Autodesk Inventor part; units mm, degrees
ref_plane "Work Plane1" through (0, 0, 20) normal (0, 0, 1) x (1, 0, 0)
ref_plane "YZ Plane" through (0, 0, 0) normal (1, 0, 0) x (0, 1, 0)
ref_plane "XZ Plane" through (0, 0, 0) normal (0, 1, 0) x (-1, 0, 0)
sketch "Sketch1" plane through (0, 0, 0) normal (0, 0, 1) x (1, 0, 0)
  line L0 (-50, 0) -> (-50, 70)
  line L1 (-50, 70) -> (-115, 70)
  line L2 (-115, 70) -> (-115, 210)
  line L3 (-115, 210) -> (-75, 210)
  line L4 (-75, 210) -> (-75, 120)
  line L5 (-75, 120) -> (75, 120)
  line L6 (75, 120) -> (75, 210)
  line L7 (75, 210) -> (115, 210)
  line L8 (115, 210) -> (115, 70)
  line L9 (115, 70) -> (50, 70)
  line L10 (50, 70) -> (50, 0)
  line L11 (50, 0) -> (-50, 0)
  point P0 (0, 0)
  point P1 (0, 120)
  point P2 (0, 0)
  dimension "d0" = 100
  dimension "d1" = 150
  dimension "d2" = 40
  dimension "d3" = 140
  dimension "d4" = 90
  dimension "d5" = 70
extrude "Extrusion1" add sketch "Sketch1" along normal blind 40
sketch "Sketch2" plane through (-50, 0, 0) normal (0, -1, 0) x (1, 0, 0)
  line L0 (0, 0) -> (0, 40)
  line L1 (100, 0) -> (100, 40)
  line L2 (0, 40) -> (100, 40)
  circle A0 centre (50, 20) radius 2.5
  point P0 (50, 0)
  dimension "d8" = 5
extrude "Extrusion2" cut sketch "Sketch2" against normal blind 40
ref_plane "Work Plane1" through (0, 0, 20) normal (0, 0, 1) x (1, 0, 0)
sketch "Sketch3" plane through (0, 0, 20) normal (0, 0, 1) x (1, 0, 0)
  line L0 (-50, 0) -> (50, 0)
  line L1 (0, 0) -> (50, 0)
  line L2 (50, 0) -> (50, -70)
  line L3 (50, -70) -> (39.0685, -70)
  line L4 (39.0685, -70) -> (39.0685, -10.9315)
  line L5 (39.0685, -10.9315) -> (0, -10.9315)
  line L6 (0, -10.9315) -> (0, 0)
  dimension "d12" = 70
  dimension "d13" = 39.0685
extrude "Extrusion3" add sketch "Sketch3" along normal blind 40
sketch "Sketch4" plane through (50, 0, 0) normal (1, 0, 0) x (0, 0, -1)
  circle A0 centre (-40, -65) radius 2.5
  line L0 (-20, -70) -> (-60, -70)
  point P0 (0, 0)
  point P1 (-40, -70)
  point P2 (-40, -70)
  dimension "d16" = 5
  dimension "d17" = 5
extrude "Extrusion4" cut sketch "Sketch4" against normal blind 40
properties part number "Robot_arm_gripper"
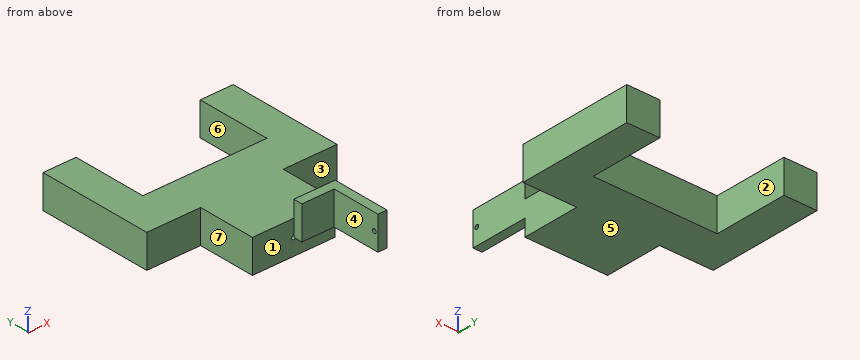
Geometry: final body of the model. Coordinates: model frame, mm. Face numbers are marked on the shaded views. A direction names the side the tool comes from. Round coordinates to 2 decimals unless told otherwise and drop trailing zeros. Loops run counter-clockwise (first coordinate to the right, second up) from the corner with the lowest first, then second, coordinate; pieces in that order, holes last. Notation, with made-up numbers: (-6.5, 55) -> (33.5, 55) arc R4 cw to (33.5, 62) -> close; hole circle Ø1 at (79, -17). An arc over 180 degrees is marked (long way). Use one line per item in the form item = value. Start each with the question number.
1) Section D-D on y = 86.5. Output: boundary loops of the cut face in (x, z), then the cut area to 3 significant figures.
2) First-contact query: P1, Ø20, axis at y = 31, z = 12, coming from the -X side; P2, Ø12, axis at x = 14.5, z = 26, coming from the -Y side; P3, Ø2, axis at y = 29.5, z = 40.5, coming from the +X side. Flat tips, straight axial feed; report the tip coordinate or a pass-through.
3) Draft query along X for the marked faces 5, 6 and 7. Return one class per face: released by +X, released by -X, zero draft, split by the parting line, or undercut.
4) Access query for the marked faces 1, 2, 3 and 4. Directions: +Z, -Z, +X, -X, +Y, -Y. A direction counts if a zero-diameter tool reaches every point of the face in a straight line with its end or side. Return the directions, or none.
5) Section C-C on x = -86. Output: boundary loops of the cut face in (y, z), then the cut area to 3 significant figures.
6) Line query: L1, parallel to Z at x = 0, y = 23.5; L2, parallel to X at y = 27, z = 20; L3, parallel to X at y = 134, z = 17. Output: solid intervals per line, ascending.
7) Section B-B on z = 10.5. Output: boundary loops of the cut face in (x, y).
8) Section A-A on y = 177.5. Output: boundary loops of the cut face in (x, z).
Response:
q1.outline = (-115, 0) -> (115, 0) -> (115, 40) -> (-115, 40) -> close
q1.area = 9,200 mm^2
q2.P1 = -50
q2.P2 = -10.93
q2.P3 = 50
q3.face_5 = zero draft
q3.face_6 = undercut
q3.face_7 = released by -X
q4.face_1 = -Z, -X, -Y
q4.face_2 = +Z, -Z, +Y
q4.face_3 = +Z, -Z, +X, -Y
q4.face_4 = +Z, -Z, -X, -Y
q5.outline = (70, 0) -> (210, 0) -> (210, 40) -> (70, 40) -> close
q5.area = 5,600 mm^2
q6.L1 = 0 to 17.5, 22.5 to 40
q6.L2 = -50 to -2.5, 2.5 to 50
q6.L3 = -115 to -75, 75 to 115
q7.outline = (-115, 70) -> (-50, 70) -> (-50, 0) -> (50, 0) -> (50, 70) -> (115, 70) -> (115, 210) -> (75, 210) -> (75, 120) -> (-75, 120) -> (-75, 210) -> (-115, 210) -> close
q8.outline = (-115, 0) -> (-75, 0) -> (-75, 40) -> (-115, 40) -> close; (75, 0) -> (115, 0) -> (115, 40) -> (75, 40) -> close
